Model file for the job. Use its own axes, mm. Give positions to 0.01 mm unless a question says otherwise; leave off trailing zeros. Loops run counter-clockwise (first coordinate to the right, second up) from the corner with the lowest first, then second, coordinate; pieces in that order, holes last. Notation, with made-up numbers: M 47.25,-12.5 L 105.25,-12.5 A15 cw 105.25,6.5 Z; hole C 80,1.5 d8. An arc over 180 degrees is marked long. Use CSV: the item, a comma, the result in double quotes. Start each with the question number.
(1) Two-plate mould, pull along X, no slides. Class faces 1 (the face through (-4, 0, 0)), 2 (the face through (53.925, -6.929, 2.465)), 3 (the face through (47.75, -9.88, 2.46)): pulls with the +X half, pulls with the -X half, needs draft (parallel to the pull), parting line crosses it, or undercut.
(2) Flat gauge pins, fed straight in: P1, Ø3, axis at y = 13.5, z = 3.5, coming from the +X side; P2, Ø6, axis at x = -10.5, y = 5, coming from the +Z side; P3, Ø2, axis at y = 7.5, z = 3.5, coming from the -X side. Where does each tip first touch, or does it go through?
(3) Slice it at D-D on y = -12. List the corners of the cut face in (x, z).
(4) Slice it at B-B on x = -25. List the corners of the cut face in (y, z), and give its area (3 significant figures).
(5) Slice it at C-C on x = 20. List the corners of the cut face in (y, z), and give its area (3 significant figures).
(6) Wall check: line 1 along X through (y, z) = (-8, 4.05); line 2 along X through (y, z) = (10, 3.4); line 3 along Y through (x, z) = (-20, 0.7). Give the ranges that are in metal, low to high. Write a range as from..to.
(7) Slice it at A-A on y = 0. List the corners of the cut face in (x, z) (3 decimals).
```python
from build123d import *

# Parameters (mm, degrees)
ESBO_O1_R                = 25.8
ESBO_O1_R_2              = 19
RESSALTO_EXTRUS_O1_DEPTH = 5


with BuildPart() as part:
    # Esboço1 → Ressalto-extrusão1 (new body)
    with BuildSketch(Plane.XY):
        with BuildLine():
            ThreePointArc((-23.915, 24), (-47.915, 0), (-23.915, -24))
            add(Edge.make_bspline(
                [(-23.915, -24), (-6.056429517, -24.659084063), (11.802140965, -28.318168126)],
                knots=[0, 0, 0, 0.74675185, 0.74675185, 0.74675185], degree=2))
            ThreePointArc((11.802140965, -28.318168126), (54.088163393, -6.18224966), (23.915, 30.8))
            Line((23.915, 30.8), (-23.915, 24))
        make_face()
        with Locations((23.915, 0)):
            Circle(ESBO_O1_R, mode=Mode.SUBTRACT)
        with Locations((-23.915, 0)):
            Circle(ESBO_O1_R_2, mode=Mode.SUBTRACT)
    extrude(amount=RESSALTO_EXTRUS_O1_DEPTH)


solid = part.part
```
Reply:
1,face 1,"needs draft"
1,face 2,"parting line crosses it"
1,face 3,"undercut"
2,P1,"stops at x = 52.28"
2,P2,"passes through"
2,P3,"stops at x = -47.02"
3,outline,"M -44.7,0 L -38.65,0 L -38.65,5 L -44.7,5 Z; M -9.18,0 L 1.08,0 L 1.08,5 L -9.18,5 Z; M 46.75,0 L 52.28,0 L 52.28,5 L 46.75,5 Z"
4,outline,"M -23.98,0 L -18.97,0 L -18.97,5 L -23.98,5 Z; M 18.97,0 L 23.98,0 L 23.98,5 L 18.97,5 Z"
4,area,"50.1 mm^2"
5,outline,"M -30.55,0 L -25.5,0 L -25.5,5 L -30.55,5 Z; M 25.5,0 L 30.24,0 L 30.24,5 L 25.5,5 Z"
5,area,"49.0 mm^2"
6,line 1,"x = -46.54..-41.15, -6.68..-0.61, 48.44..53.66"
6,line 2,"x = -45.73..-40.07, -7.76..0.13, 47.7..53.05"
6,line 3,"y = -24.18..-18.59, 18.59..24.56"
7,outline,"M -47.915,0 L -42.915,0 L -42.915,5 L -47.915,5 Z; M -4.915,0 L -1.885,0 L -1.885,5 L -4.915,5 Z; M 49.715,0 L 54.715,0 L 54.715,5 L 49.715,5 Z"
